Autodesk Inventor part; units mm, degrees
ref_plane "YZ Plane" through (0, 0, 0) normal (1, 0, 0) x (0, 1, 0)
ref_plane "XZ Plane" through (0, 0, 0) normal (0, 1, 0) x (-1, 0, 0)
ref_plane "XY Plane" through (0, 0, 0) normal (0, 0, 1) x (1, 0, 0)
sketch "Sketch1" plane through (0, 0, 0) normal (0, 1, 0) x (-1, 0, 0)
  line L0 (1.6, -12.1429) -> (-1.6, -12.1429)
  line L1 (-1.6, -12.1429) -> (-11.3161, 4.6858)
  line L2 (-11.3161, 4.6858) -> (-9.7161, 7.4571)
  line L3 (-9.7161, 7.4571) -> (9.7161, 7.4571)
  line L4 (9.7161, 7.4571) -> (11.3161, 4.6858)
  line L5 (11.3161, 4.6858) -> (1.6, -12.1429)
  circle A0 centre (0, 0) radius 7.4571 construction
  dimension "d0" = 19.6
  dimension "d1" = 3.2
  dimension "d4" = 14.9142
extrude "Extrusion1" add sketch "Sketch1" along normal mid plane 30.6
properties part number "FactionSpecial_Council_CommandToken" material "ABS Plastic"
Geometry check sheet. Reference: the model listing, model coordinates, mm. Give positions to 0.01 mm unless a question says otherwise; leave off trailing zeros. Write each loop counter-clockwise with the first axis right and the second up, starting at its lowest first coordinate (ties: lowest second). Pieces come first, ordered by that corner, then holes. Notation, with made-up numbers: M 54.5,59.25 L 73.5,59.25 A23 ccw 73.5,68.25 Z; hole C 37.5,81 d4. An arc over 180 degrees is marked long. One line per question, with ' | ' between items.
1. Cross-section at B-B (x = 6). Enter the section's corners in (y, z).
Ans:
outline: M -15.3,-4.52 L 15.3,-4.52 L 15.3,7.46 L -15.3,7.46 Z
2. Cross-section at C-C (z = 2.5). Enter the section's corners in (x, y).
Ans:
outline: M -10.05,-15.3 L 10.05,-15.3 L 10.05,15.3 L -10.05,15.3 Z
3. Cross-section at A-A (y = -8). Enter the section's corners in (x, z).
Ans:
outline: M -11.32,4.69 L -1.6,-12.14 L 1.6,-12.14 L 11.32,4.69 L 9.72,7.46 L -9.72,7.46 Z
4. Scan lines: line 1 along Z through (x, y) = (3, 2); line 2 along X through (y, z) = (10.5, -11.5); line 3 along Z through (x, y) = (9.5, 10). Record each from-to range of solid material in increasing order. Write a range as from..to.
Ans:
line 1: -9.72..7.46 | line 2: -1.97..1.97 | line 3: 1.54..7.46
